Verification items for the finished model (mm, model axes). A direction names the side the tool comes from. Give positions to 0.01 mm unless a question says otherwise; leave off trailing zeros. Loops run counter-clockwise (first coordinate to the right, second up) from the corner with the lowest first, then second, coordinate; pieces in that order, holes last. Notation, with made-up numbers: (51, 33) - (65, 33) arc R25 ccw to (65, 54) - close; hole circle Ø11 at (-16, 13). An arc over 180 degrees is marked (long way). One line per question, with ' | ' between items. Start each with the question number.
1. Thickness scan on line 1 along X through (y, z) = (-2, 81); line 2 along Y through (x, z) = (40.25, 87); line 3 along Y through (x, z) = (41.5, 74). Record the ranges inside material, lowest first. Write a range as from..to.
2. Depth check by flat-ended pin: pin 1 Ø1.2 at (x, z) = (24.5, 69) entering from +Y; pin 2 Ø5 at (x, z) = (34.5, 44.5) entering from -Y; pin 3 Ø4 at (x, y) = (33.68, 5.26) entering from +Z; pin 4 Ø1.3 at (y, z) = (4.5, 27.5) entering from +X. Enter the tip coordinate at first touch or a pass-through.
3. Section check B-B, the plane y = 4. Enter the section's corners in (x, z).
4. Mould release check, pull along Y, two halves, no side actions. Record for faces 1 (the face through (38.243, -0.279, 49.3)), 2 (the face through (23.682, 11, 49)), 3 (the face through (38, -2.935, 49)), 4 (the face through (40, -4.735, 49)): +Y half, -Y half, draft (parallel to the pull), parting line (faces both ways), or undercut.
5. Tool access check on faces 5 (the face through (38.27, 10.84, 49.3)), 6 (the face through (29.782, 5, 49)), 7 (the face through (34, 9.165, 49)), 8 (the face through (34, 1.365, 49)). Record the directions out of +Z, -Z, +X, -X, +Y, -Y that give a thin tool (end or side, any length) a straight path to the whole face; none if there is none.
6. Section check A-A, the plane x = 33.75. Enter the section's corners in (y, z), then the cut area to 3 significant figures.
from build123d import *

# Parameters (mm, degrees)
F0_R     = 2.5
F1_DEPTH = 100


with BuildPart() as f1:
    # F0 (on Top) → F1 (new body)
    with BuildSketch(Plane.XY):
        with BuildLine():
            Line((30.582384, 13.664589), (30.582384, 14.764589))
            Line((30.582384, 14.764589), (30.082384, 15.264589))
            Line((30.082384, 15.264589), (25.182384, 15.264589))
            ThreePointArc((25.182384, 15.264589), (24.616801, 15.153875), (24.134708, 14.838077))
            ThreePointArc((24.134708, 14.838077), (24.121724, 14.825249), (24.108896, 14.812265))
            ThreePointArc((24.108896, 14.812265), (23.793098, 14.330172), (23.682384, 13.764589))
            Line((23.682384, 13.764589), (23.682384, 8.864589))
            Line((23.682384, 8.864589), (24.182384, 8.364589))
            Line((24.182384, 8.364589), (25.282384, 8.364589))
            ThreePointArc((25.282384, 8.364589), (25.423805, 8.423168), (25.482384, 8.564589))
            Line((25.482384, 8.564589), (25.482384, 10.564589))
            ThreePointArc((25.482384, 10.564589), (25.540962, 10.70601), (25.682384, 10.764589))
            Line((25.682384, 10.764589), (27.006344, 10.764589))
            ThreePointArc((27.006344, 10.764589), (27.07742, 10.751533), (27.139217, 10.714071))
            Line((27.139217, 10.714071), (29.111111, 8.961276))
            ThreePointArc((29.111111, 8.961276), (29.606864, 8.285769), (29.782384, 7.466457))
            Line((29.782384, 7.466457), (29.782384, 5.264589))
            Line((29.782384, 5.264589), (29.782384, 3.062721))
            ThreePointArc((29.782384, 3.062721), (29.606864, 2.243409), (29.111111, 1.567903))
            Line((29.111111, 1.567903), (27.139217, -0.184893))
            ThreePointArc((27.139217, -0.184893), (27.07742, -0.222355), (27.006344, -0.235411))
            Line((27.006344, -0.235411), (25.682384, -0.235411))
            ThreePointArc((25.682384, -0.235411), (25.540962, -0.176832), (25.482384, -0.035411))
            Line((25.482384, -0.035411), (25.482384, 1.964589))
            ThreePointArc((25.482384, 1.964589), (25.423805, 2.10601), (25.282384, 2.164589))
            Line((25.282384, 2.164589), (24.182384, 2.164589))
            Line((24.182384, 2.164589), (23.682384, 1.664589))
            Line((23.682384, 1.664589), (23.682384, -3.235411))
            ThreePointArc((23.682384, -3.235411), (23.793098, -3.800994), (24.108896, -4.283086))
            ThreePointArc((24.108896, -4.283086), (24.121724, -4.296071), (24.134708, -4.308899))
            ThreePointArc((24.134708, -4.308899), (24.616801, -4.624697), (25.182384, -4.735411))
            Line((25.182384, -4.735411), (30.082384, -4.735411))
            Line((30.082384, -4.735411), (30.582384, -4.235411))
            Line((30.582384, -4.235411), (30.582384, -3.135411))
            ThreePointArc((30.582384, -3.135411), (30.523805, -2.99399), (30.382384, -2.935411))
            Line((30.382384, -2.935411), (28.382384, -2.935411))
            ThreePointArc((28.382384, -2.935411), (28.240962, -2.876832), (28.182384, -2.735411))
            Line((28.182384, -2.735411), (28.182384, -1.411451))
            ThreePointArc((28.182384, -1.411451), (28.195439, -1.340375), (28.232902, -1.278578))
            Line((28.232902, -1.278578), (29.985697, 0.693317))
            ThreePointArc((29.985697, 0.693317), (30.661204, 1.189069), (31.480516, 1.364589))
            Line((31.480516, 1.364589), (33.682384, 1.364589))
            Line((33.682384, 1.364589), (35.884252, 1.364589))
            ThreePointArc((35.884252, 1.364589), (36.703564, 1.189069), (37.37907, 0.693317))
            Line((37.37907, 0.693317), (39.131866, -1.278578))
            ThreePointArc((39.131866, -1.278578), (39.169328, -1.340375), (39.182384, -1.411451))
            Line((39.182384, -1.411451), (39.182384, -2.735411))
            ThreePointArc((39.182384, -2.735411), (39.123805, -2.876832), (38.982384, -2.935411))
            Line((38.982384, -2.935411), (36.982384, -2.935411))
            ThreePointArc((36.982384, -2.935411), (36.840962, -2.99399), (36.782384, -3.135411))
            Line((36.782384, -3.135411), (36.782384, -4.235411))
            Line((36.782384, -4.235411), (37.282384, -4.735411))
            Line((37.282384, -4.735411), (42.182384, -4.735411))
            ThreePointArc((42.182384, -4.735411), (42.747967, -4.624697), (43.230059, -4.308899))
            ThreePointArc((43.230059, -4.308899), (43.243044, -4.296071), (43.255872, -4.283086))
            ThreePointArc((43.255872, -4.283086), (43.57167, -3.800994), (43.682384, -3.235411))
            Line((43.682384, -3.235411), (43.682384, 1.664589))
            Line((43.682384, 1.664589), (43.182384, 2.164589))
            Line((43.182384, 2.164589), (42.082384, 2.164589))
            ThreePointArc((42.082384, 2.164589), (41.940962, 2.10601), (41.882384, 1.964589))
            Line((41.882384, 1.964589), (41.882384, -0.035411))
            ThreePointArc((41.882384, -0.035411), (41.823805, -0.176832), (41.682384, -0.235411))
            Line((41.682384, -0.235411), (40.358424, -0.235411))
            ThreePointArc((40.358424, -0.235411), (40.287348, -0.222355), (40.225551, -0.184893))
            Line((40.225551, -0.184893), (38.253656, 1.567903))
            ThreePointArc((38.253656, 1.567903), (37.757904, 2.243409), (37.582384, 3.062721))
            Line((37.582384, 3.062721), (37.582384, 5.264589))
            Line((37.582384, 5.264589), (37.582384, 7.466457))
            ThreePointArc((37.582384, 7.466457), (37.757904, 8.285769), (38.253656, 8.961276))
            Line((38.253656, 8.961276), (40.225551, 10.714071))
            ThreePointArc((40.225551, 10.714071), (40.287348, 10.751533), (40.358424, 10.764589))
            Line((40.358424, 10.764589), (41.682384, 10.764589))
            ThreePointArc((41.682384, 10.764589), (41.823805, 10.70601), (41.882384, 10.564589))
            Line((41.882384, 10.564589), (41.882384, 8.564589))
            ThreePointArc((41.882384, 8.564589), (41.940962, 8.423168), (42.082384, 8.364589))
            Line((42.082384, 8.364589), (43.182384, 8.364589))
            Line((43.182384, 8.364589), (43.682384, 8.864589))
            Line((43.682384, 8.864589), (43.682384, 13.764589))
            ThreePointArc((43.682384, 13.764589), (43.57167, 14.330172), (43.255872, 14.812265))
            ThreePointArc((43.255872, 14.812265), (43.243044, 14.825249), (43.230059, 14.838077))
            ThreePointArc((43.230059, 14.838077), (42.747967, 15.153875), (42.182384, 15.264589))
            Line((42.182384, 15.264589), (37.282384, 15.264589))
            Line((37.282384, 15.264589), (36.782384, 14.764589))
            Line((36.782384, 14.764589), (36.782384, 13.664589))
            ThreePointArc((36.782384, 13.664589), (36.840962, 13.523168), (36.982384, 13.464589))
            Line((36.982384, 13.464589), (38.982384, 13.464589))
            ThreePointArc((38.982384, 13.464589), (39.123805, 13.40601), (39.182384, 13.264589))
            Line((39.182384, 13.264589), (39.182384, 11.940629))
            ThreePointArc((39.182384, 11.940629), (39.169328, 11.869553), (39.131866, 11.807756))
            Line((39.131866, 11.807756), (37.37907, 9.835861))
            ThreePointArc((37.37907, 9.835861), (36.703564, 9.340109), (35.884252, 9.164589))
            Line((35.884252, 9.164589), (33.682384, 9.164589))
            Line((33.682384, 9.164589), (31.480516, 9.164589))
            ThreePointArc((31.480516, 9.164589), (30.661204, 9.340109), (29.985697, 9.835861))
            Line((29.985697, 9.835861), (28.232902, 11.807756))
            ThreePointArc((28.232902, 11.807756), (28.195439, 11.869553), (28.182384, 11.940629))
            Line((28.182384, 11.940629), (28.182384, 13.264589))
            ThreePointArc((28.182384, 13.264589), (28.240962, 13.40601), (28.382384, 13.464589))
            Line((28.382384, 13.464589), (30.382384, 13.464589))
            ThreePointArc((30.382384, 13.464589), (30.523805, 13.523168), (30.582384, 13.664589))
        make_face()
        with Locations((33.682384, 5.264589)):
            Circle(F0_R, mode=Mode.SUBTRACT)
    extrude(amount=F1_DEPTH)


solid = f1.part
Results list:
1) line 1: 23.68..28.18, 39.18..43.68 | line 2: -4.74..-0.2, 10.73..15.26 | line 3: -4.74..-0.24, 10.76..15.26
2) pin 1: y = 15.26 | pin 2: y = -4.45 | pin 3: through | pin 4: x = 37.58
3) outline: (29.78, 0) - (31.53, 0) - (31.53, 100) - (29.78, 100) - close; (35.84, 0) - (37.58, 0) - (37.58, 100) - (35.84, 100) - close
4) face 1: undercut | face 2: draft | face 3: undercut | face 4: -Y half
5) face 5: +Z, -Z | face 6: +Z, -Z, -X | face 7: +Z, -Z, +Y | face 8: +Z, -Z, -Y
6) outline: (1.36, 0) - (2.77, 0) - (2.77, 100) - (1.36, 100) - close; (7.76, 0) - (9.16, 0) - (9.16, 100) - (7.76, 100) - close | area: 280 mm²
